Verification items for this drawing (mm, ordinates from the low corner). A direction names the side the tool comes from. Coordinates: 2 decimals unless noted, no trailing zeros. Order: outer loops, then holes, each group sorted by start corner. A loop starts at its lowest first (then second) coordinate and runs counter-clockwise, first axis right, second up. Notation, with made-up numbers: M 46,-6.75 L 57,-6.75 A18 cw 57,3.25 Z; hole C -38,-15.5 d4. An arc over 180 degrees is marked long. Use CSV: the item, a comma, the result in double quotes. Start each with the question number.
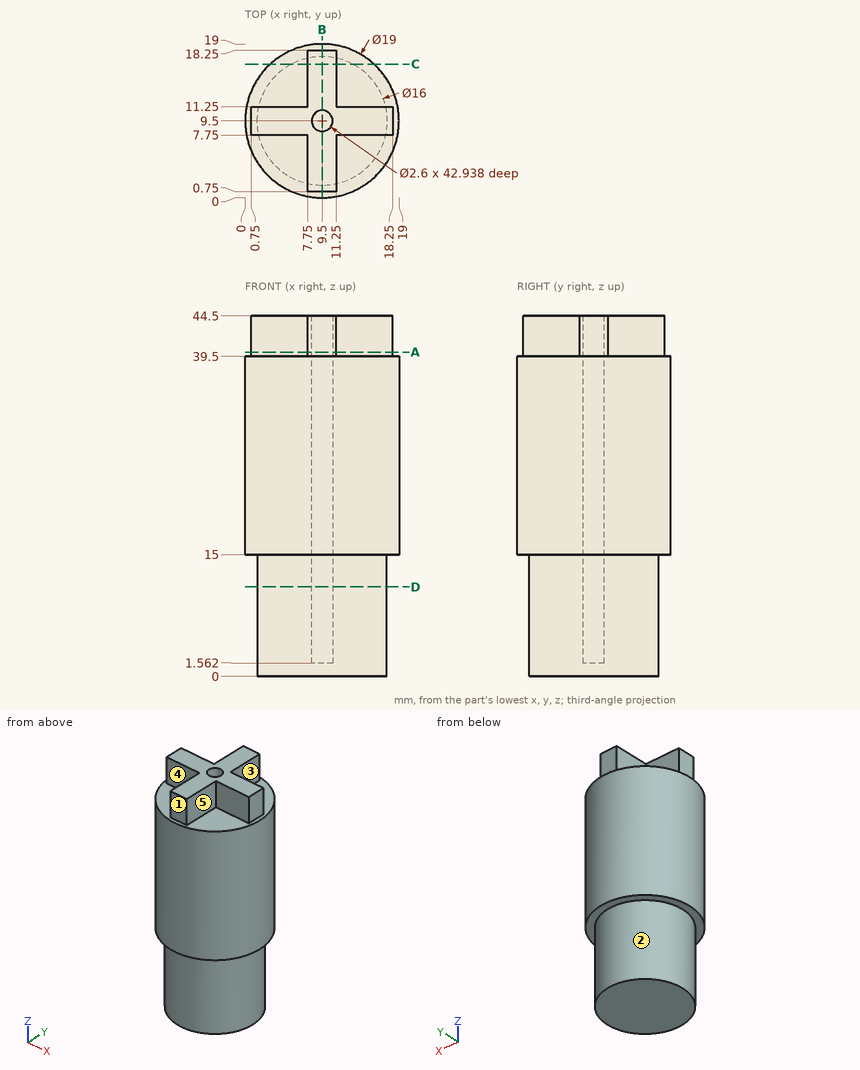
1) Set-up check for the marked faces 1, 2, 3, 4 and 5: record each of +Z, -Z, +X, -X, +Y, -Y from which the full face is reachable in a straight line by a thin tool's end or side.
2) Material ranges on line 1 along Y through (x, z) = (9.5, 36); line 2 along Y through (x, z) = (9.5, 13.5); line 3 along Z through (x, y) = (18, 11), recorded low to high.
3) Gauge pin test, flat ends, axial feed: P1, Ø4, axis at x = 6, z = 42, coming from the -Y side; P2, Ø10, axis at y = 16, z = 19, coming from the -X side; P3, Ø4, axis at x = 15.5, z = 35, coming from the +Y side. Record the tip position at first contact, or that the pin passes through.
4) Section check D-D on z = 11. Record the boundary of the cut face in (x, y), then the cut area to 3 significant figures.
5) Section check C-C on y = 16.5. Record the boundary of the cut face in (x, z).
6) Section check B-B on x = 9.5. Record the boundary of the cut face in (y, z).
7) Section check A-A on z = 40. Record the boundary of the cut face in (x, y), then the cut area to 3 significant figures.
Results are:
1,face 1,"+Z, +X, -X, -Y"
1,face 2,"-Z"
1,face 3,"+Z, +X, +Y"
1,face 4,"+Z, -X, -Y"
1,face 5,"+Z, +X, -Y"
2,line 1,"y = 0 to 8.2, 10.8 to 19"
2,line 2,"y = 1.5 to 8.2, 10.8 to 17.5"
2,line 3,"z = 15 to 44.5"
3,P1,"stops at y = 0.75"
3,P2,"stops at x = 0.12"
3,P3,"stops at y = 18.12"
4,outline,"C 9.5,9.5 d16; hole C 9.5,9.5 d2.6"
4,area,"196 mm²"
5,outline,"M 3.08,15 L 5.63,15 L 5.63,0 L 13.37,0 L 13.37,15 L 15.92,15 L 15.92,39.5 L 11.25,39.5 L 11.25,44.5 L 7.75,44.5 L 7.75,39.5 L 3.08,39.5 Z"
6,outline,"M 0,15 L 1.5,15 L 1.5,0 L 17.5,0 L 17.5,15 L 19,15 L 19,39.5 L 18.25,39.5 L 18.25,44.5 L 10.8,44.5 L 10.8,1.56 L 8.2,1.56 L 8.2,44.5 L 0.75,44.5 L 0.75,39.5 L 0,39.5 Z"
7,outline,"M 0.75,7.75 L 7.75,7.75 L 7.75,0.75 L 11.25,0.75 L 11.25,7.75 L 18.25,7.75 L 18.25,11.25 L 11.25,11.25 L 11.25,18.25 L 7.75,18.25 L 7.75,11.25 L 0.75,11.25 Z; hole C 9.5,9.5 d2.6"
7,area,"105 mm²"
